Design review of the part built by this model. Coordinates are the model's own, in mm. Face numbers are marked on the shaded views. A direction names the side the tool comes from. Coordinates: 2 decimals unless noted, no trailing zeros. Loops run counter-clockwise (first coordinate to the right, second up) from the corner with the lowest first, then second, coordinate; pieces in that order, holes last.
Q1. For P1, Ø5, axis at x = -46.5, y = 15, coming from the -Z side; P2, Ø4.5, axis at y = -15.5, z = 38, coming from the +X side; P3, Ø2, axis at y = -14.5, z = 37.5, coming from the -X side; P4, Ø3.5, axis at x = -42.5, z = 7.5, coming from the -Y side, all flat-tipped, find the tip position at first contact; note any pin that passes through.
Q2. Draft analysis for pull direction X (two halves, no side actions). For the marked faces 1, 2 and 3, state which applies: released by +X, released by -X, zero draft, split by the parting line, or undercut.
Q3. Wall thickness on probe 1 along X at (y, z) = (-17, 50); probe 2 along Y at (x, z) = (-23, 22); probe 3 along Z at (x, y) = (-29.5, 12): over which ranges is each line inside the solid? List them lowest first.
Q4. Add section A-A on x = 0. Give the boundary of the cut face in (y, z), and give its area (3 significant figures).
Q5. Add section B-B on z = 41. Give the boundary of the cut face in (x, y), and give its area (3 significant figures).
Q6. Machinability: for the marked faces 4 and 5, which of the approach directions +Z, -Z, +X, -X, +Y, -Y give a long, thin tool a straight path to every point of the face, cutting with its end or side? Answer none if there is none.
```python
from build123d import *

# Parameters (mm, degrees)
ESQUISSE1_W             = 130
ESQUISSE1_H             = 40
BOSS_EXTRU_1_DEPTH      = 10
ESQUISSE2_R             = 15
BOSS_EXTRU_2_DEPTH      = 10
ENL_V_MAT_EXTRU_1_DEPTH = 98.59610648
ESQUISSE4_W             = 20
ESQUISSE4_H             = 3
ENL_V_MAT_EXTRU_2_DEPTH = 111.566721937
CONG_5_START            = -20
CONG_5_DEPTH            = 40
CONG_5_START_2          = -4.421e-06
CONG_5_2_DEPTH          = 3.000004421
CHANFREIN1_SIZE         = 6
CONG_6_R                = 3


with BuildPart() as part:
    # Esquisse1 → Boss.-Extru.1 (new body)
    with BuildSketch(Plane.XY):
        Rectangle(ESQUISSE1_W, ESQUISSE1_H)
    extrude(amount=BOSS_EXTRU_1_DEPTH)

    # Esquisse2 → Boss.-Extru.2 (add)
    with BuildSketch(Plane.XZ.offset(20)):
        with BuildLine():
            Line((-30, 0), (-30, 50))
            ThreePointArc((-30, 50), (0, 80), (30, 50))
            Line((30, 50), (30, 0))
            Line((30, 0), (-30, 0))
        make_face()
        with Locations(Location((0, 50, 0), (0, 0, 270))):
            Circle(ESQUISSE2_R, mode=Mode.SUBTRACT)
    extrude(amount=-BOSS_EXTRU_2_DEPTH)

    # Esquisse3 → Enlèv. mat.-Extru.1 (cut, through all)
    with BuildSketch(Plane.XY.offset(10)):
        with BuildLine():
            Line((38, 8), (52, 8))
            ThreePointArc((52, 8), (55, 5), (52, 2))
            Line((52, 2), (38, 2))
            ThreePointArc((38, 2), (35, 5), (38, 8))
        make_face()
    enl_v_mat_extru_1 = extrude(amount=-ENL_V_MAT_EXTRU_1_DEPTH, mode=Mode.SUBTRACT)

    # Symétrie1: Enlèv. mat.-Extru.1 across plane
    add(enl_v_mat_extru_1.mirror(Plane(origin=(0, 0, 0), x_dir=(0, 0, 1), z_dir=(1, 0, 0))), mode=Mode.SUBTRACT)

    # Esquisse4 → Enlèv. mat.-Extru.2 (cut, through all)
    with BuildSketch(Plane(origin=(0, 20, 0), x_dir=(1, 0, 0), z_dir=(0, 1, 0))):
        with Locations((45, -1.5)):
            Rectangle(ESQUISSE4_W, ESQUISSE4_H)
    enl_v_mat_extru_2 = extrude(amount=-ENL_V_MAT_EXTRU_2_DEPTH, mode=Mode.SUBTRACT)

    # Congé5: read off the stored shape, not the designer's step
    # Congé5 outline → Congé5 (add)
    with BuildSketch(Plane(origin=(0, 0, 0), x_dir=(1, 0, 0), z_dir=(0, 1, 0)).offset(CONG_5_START)):
        with BuildLine():
            Line((55, -3), (55.000002552, 4.421e-06))
            ThreePointArc((55.000002552, 4.421e-06), (52.803849788, -2.196151147), (49.803847577, -3))
            Line((49.803847577, -3), (55, -3))
        make_face()
        with BuildLine():
            Line((35, -3), (40.196152423, -3))
            ThreePointArc((40.196152423, -3), (37.196152423, -2.196152423), (35, 0))
            Line((35, 0), (35, -3))
        make_face()
    cong_5 = extrude(amount=CONG_5_DEPTH)

    # Cong_5 2 outline → Cong_5 2 (cut)
    with BuildSketch(Plane.XY.offset(CONG_5_START_2)):
        with BuildLine():
            Line((52, 8), (38, 8))
            ThreePointArc((38, 8), (35, 5), (38, 2))
            Line((38, 2), (52, 2))
            ThreePointArc((52, 2), (55, 5), (52, 8))
        make_face()
    cong_5_2 = extrude(amount=CONG_5_2_DEPTH, mode=Mode.SUBTRACT)

    # Symétrie2: Enlèv. mat.-Extru.2, Congé5, Cong_5 2 across plane
    add(enl_v_mat_extru_2.mirror(Plane(origin=(0, 0, 0), x_dir=(0, 0, 1), z_dir=(1, 0, 0))), mode=Mode.SUBTRACT)
    add(cong_5.mirror(Plane(origin=(0, 0, 0), x_dir=(0, 0, 1), z_dir=(1, 0, 0))))
    add(cong_5_2.mirror(Plane(origin=(0, 0, 0), x_dir=(0, 0, 1), z_dir=(1, 0, 0))), mode=Mode.SUBTRACT)

    # Chanfrein1
    chanfrein1_edges = [part.edges().sort_by_distance(p)[0] for p in [
        (65, -20, 5),
        (-65, -20, 5),
        (-65, 20, 5),
        (65, 20, 5),
    ]]
    chamfer(chanfrein1_edges, length=CHANFREIN1_SIZE)

    # Congé6
    cong_6_edges = [part.edges().sort_by_distance(p)[0] for p in [
        (44.5, -20, 10),
        (65, 0, 10),
        (-44.5, -20, 10),
        (0, 20, 10),
        (-65, 0, 10),
        (-62, 17, 10),
        (62, 17, 10),
        (-62, -17, 10),
        (62, -17, 10),
        (-30, -10, 30),
        (-30, -15, 10),
        (0, -10, 80),
        (30, -15, 10),
        (30, -10, 30),
        (0, -10, 10),
        (30, -20, 30),
        (0, -20, 80),
        (-30, -20, 30),
    ]]
    fillet(cong_6_edges, radius=CONG_6_R)


solid = part.part
```
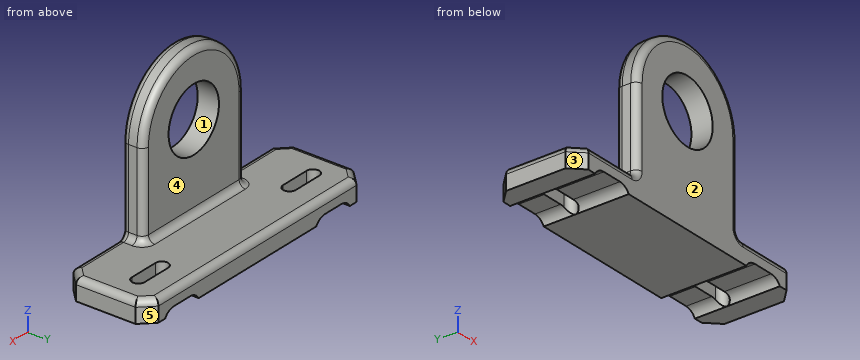
Entries:
1. P1: stops at z = 3
1. P2: stops at x = 30
1. P3: stops at x = -30
1. P4: stops at y = -20
2. face 1: undercut
2. face 2: zero draft
2. face 3: released by -X
3. probe 1: x = -30 to -15, 15 to 30
3. probe 2: y = -20 to -10
3. probe 3: z = 0 to 10
4. outline: (-20, 0) - (20, 0) - (20, 7) arc R3 ccw to (17, 10) - (-7, 10) arc R3 cw to (-10, 13) - (-10, 35) - (-20, 35) - close; (-20, 65) - (-10, 65) - (-10, 77) arc R3 ccw to (-13, 80) - (-17, 80) arc R3 ccw to (-20, 77) - close
4. area: 796 mm2
5. outline: (-30, -17) arc R3 ccw to (-27, -20) - (-12, -20) - (-12, -10) - (-27, -10) arc R3 ccw to (-30, -13) - close; (12, -20) - (27, -20) arc R3 ccw to (30, -17) - (30, -13) arc R3 ccw to (27, -10) - (12, -10) - close
5. area: 352 mm2
6. face 4: +Z, +X, -X, +Y
6. face 5: +Z, -Z, +X, +Y
